```python
from build123d import *

# Parameters (mm, degrees)
BOX018_W               = 5.8
BOX018_H               = 8.7
BOX018_DEPTH           = 4
BOX019_W               = 1.6
BOX019_H               = 3.6
BOX019_DEPTH           = 8.5
BOX016_W               = 3.8
BOX016_H               = 8.5
BOX016_DEPTH           = 9.3
BOX017_W               = 7
BOX017_H               = 12
BOX017_DEPTH           = 9.2
CUT002_ROLL_ANGLE      = 180
CUT002_PLACEMENT_ANGLE = 90
BOX010_W               = 8
BOX010_H               = 3
BOX010_DEPTH           = 2
BOX009_W               = 8
BOX009_H               = 2
BOX009_DEPTH           = 2
BOX011_W               = 8
BOX011_H               = 2
BOX011_DEPTH           = 2
BOX012_W               = 8
BOX012_H               = 3
BOX012_DEPTH           = 2
BOX013_W               = 8
BOX013_H               = 32
BOX013_DEPTH           = 2
BOX014_W               = 15.2
BOX014_H               = 6.6
BOX014_DEPTH           = 4.5
BOX015_W               = 19
BOX015_H               = 10
BOX015_DEPTH           = 5
CUT001_ROLL_ANGLE      = 180
CUT001_PLACEMENT_ANGLE = 90


with BuildPart() as cube017:
    # Box018 → Box018 (new body)
    with BuildSketch(Plane.XY):
        with Locations((2.9, 4.35)):
            Rectangle(BOX018_W, BOX018_H)
    extrude(amount=BOX018_DEPTH)


with BuildPart() as cube018:
    # Box019 → Box019 (new body)
    with BuildSketch(Plane(origin=(1.1, 2.5, 1), x_dir=(1, 0, 0), z_dir=(0, 0, 1))):
        with Locations((0.8, 1.8)):
            Rectangle(BOX019_W, BOX019_H)
    extrude(amount=BOX019_DEPTH)


with BuildPart() as fusion008:
    # Box016 → Box016 (new body)
    with BuildSketch(Plane.XY):
        with Locations((1.9, 4.25)):
            Rectangle(BOX016_W, BOX016_H)
    extrude(amount=BOX016_DEPTH)

    # Fusion008: union Cube017, Cube018
    add(cube017.part)
    add(cube018.part)


with BuildPart() as cut002:
    # Box017 → Box017 (new body)
    with BuildSketch(Plane(origin=(-1.6, -1.65, -0.6), x_dir=(1, 0, 0), z_dir=(0, 0, 1))):
        with Locations((3.5, 6)):
            Rectangle(BOX017_W, BOX017_H)
    extrude(amount=BOX017_DEPTH)

    # Cut002: cut Fusion008
    add(fusion008.part, mode=Mode.SUBTRACT)


with BuildPart() as cut002_1:
    # Cut002 roll: moved
    add(cut002.part.rotate(Axis((0, 0, 0), (1, 0, 0)), CUT002_ROLL_ANGLE))


with BuildPart() as cut002_2:
    # Cut002 placement: moved
    add(cut002_1.part.moved(Location((-0.35, -24.6, 1))).rotate(Axis((-0.35, -24.6, 1), (0, 0, 1)), CUT002_PLACEMENT_ANGLE))


with BuildPart() as cube010:
    # Box010 → Box010 (new body)
    with BuildSketch(Plane(origin=(0, 2.7, 5), x_dir=(1, 0, 0), z_dir=(0, 0, 1))):
        with Locations((4, 1.5)):
            Rectangle(BOX010_W, BOX010_H)
    extrude(amount=BOX010_DEPTH)


with BuildPart() as fusion006:
    # Box009 → Box009 (new body)
    with BuildSketch(Plane(origin=(0, 3.75, 3.5), x_dir=(1, 0, 0), z_dir=(0, 0, 1))):
        with Locations((4, 1)):
            Rectangle(BOX009_W, BOX009_H)
    extrude(amount=BOX009_DEPTH)

    # Fusion006: union Cube010
    add(cube010.part)


with BuildPart() as cube011:
    # Box011 → Box011 (new body)
    with BuildSketch(Plane(origin=(0, -26.3, 3.5), x_dir=(1, 0, 0), z_dir=(0, 0, 1))):
        with Locations((4, 1)):
            Rectangle(BOX011_W, BOX011_H)
    extrude(amount=BOX011_DEPTH)


with BuildPart() as fusion005:
    # Box012 → Box012 (new body)
    with BuildSketch(Plane(origin=(0, -26.3, 5), x_dir=(1, 0, 0), z_dir=(0, 0, 1))):
        with Locations((4, 1.5)):
            Rectangle(BOX012_W, BOX012_H)
    extrude(amount=BOX012_DEPTH)

    # Fusion005: union Cube011
    add(cube011.part)


with BuildPart() as fusion007:
    # Box013 → Box013 (new body)
    with BuildSketch(Plane(origin=(0, -26.3, 1.5), x_dir=(1, 0, 0), z_dir=(0, 0, 1))):
        with Locations((4, 16)):
            Rectangle(BOX013_W, BOX013_H)
    extrude(amount=BOX013_DEPTH)

    # Fusion007: union Fusion006, Fusion005
    add(fusion006.part)
    add(fusion005.part)


with BuildPart() as converter:
    # Box014 → Box014 (new body)
    with BuildSketch(Plane.XY):
        with Locations((7.6, 3.3)):
            Rectangle(BOX014_W, BOX014_H)
    extrude(amount=BOX014_DEPTH)


with BuildPart() as fusion009:
    # Box015 → Box015 (new body)
    with BuildSketch(Plane(origin=(-1.7, -1.5, -1), x_dir=(1, 0, 0), z_dir=(0, 0, 1))):
        with Locations((9.5, 5)):
            Rectangle(BOX015_W, BOX015_H)
    extrude(amount=BOX015_DEPTH)

    # Cut001: cut converter
    add(converter.part, mode=Mode.SUBTRACT)


with BuildPart() as fusion009_1:
    # Cut001 roll: moved
    add(fusion009.part.rotate(Axis((0, 0, 0), (1, 0, 0)), CUT001_ROLL_ANGLE))


with BuildPart() as fusion009_2:
    # Cut001 placement: moved
    add(fusion009_1.part.moved(Location((0.5, -11.7, 0.5))).rotate(Axis((0.5, -11.7, 0.5), (0, 0, 1)), CUT001_PLACEMENT_ANGLE))

    # Fusion009: union Cut002, Fusion007
    add(cut002_2.part)
    add(fusion007.part)


solid = fusion009_2.part
```
For this review, take the finished solid that the model builds, in its own axes (mm). A direction names the side the tool comes from. Coordinates: 2 decimals unless noted, no trailing zeros. Write each loop counter-clockwise with the first axis right and the second up, starting at its lowest first coordinate (ties: lowest second). Pieces come first, ordered by that corner, then holes. Notation, with made-up numbers: (6, 2.25) -> (64, 2.25) arc R30 ccw to (64, 25.25) -> close; hole circle Ø5 at (-22, -22). An arc over 180 degrees is marked (long way). Put each result on its own line as item: value.
Q1. Clearance check with flat-ended pins moving along their axes: pin 1 Ø2 at (x, z) = (4, -1.5) entering from +Y; pin 2 Ø1.2 at (y, z) = (-7.5, -1) entering from +X; pin 3 Ø8 at (y, z) = (-13, -4) entering from -X. State where each tip first meets the part, or that it passes through.
From the geometry:
pin 1: stops at y = 5.6
pin 2: stops at x = 9
pin 3: stops at x = -1
Q2. Take a section at B-B, the plane z = -0.5. State the section outline as (x, y) points, then the cut area to 3 significant figures.
From the geometry:
outline: (-2, -26.2) -> (10, -26.2) -> (10, -19.2) -> (8.35, -19.2) -> (8.35, -24.6) -> (-0.35, -24.6) -> (-0.35, -19.2) -> (-2, -19.2) -> close; (-1, -13.4) -> (9, -13.4) -> (9, 5.6) -> (-1, 5.6) -> close; hole (0.5, -11.7) -> (7.1, -11.7) -> (7.1, 3.5) -> (0.5, 3.5) -> close
area: 127 mm2
Q3. Take a section at D-D, the plane y = -5. State the section outline as (x, z) points, then the cut area to 3 significant figures.
From the geometry:
outline: (-1, -3.5) -> (0.5, -3.5) -> (0.5, 0.5) -> (7.1, 0.5) -> (7.1, -3.5) -> (9, -3.5) -> (9, 1.5) -> (8, 1.5) -> (8, 3.5) -> (0, 3.5) -> (0, 1.5) -> (-1, 1.5) -> close
area: 39.6 mm2
Q4. Take a section at C-C, the plane z = 4.5. State the section outline as (x, y) points, then the cut area to 3 significant figures.
From the geometry:
outline: (0, -26.3) -> (8, -26.3) -> (8, -24.3) -> (0, -24.3) -> close; (0, 3.75) -> (8, 3.75) -> (8, 5.75) -> (0, 5.75) -> close
area: 32.0 mm2
Q5. Tool access review of faces 5 (the flat face through (-0.35, -23, -3)), 6 (the flat face through (7.4, -4, -3.5)), 7 (the flat face through (4, 3, 5)), 8 (the flat face through (0.5, -4, -1)), 9 (the flat face through (-1, -4, -1)): name each direction out of +Z, -Z, +X, -X, +Y, -Y from which nothing blocks a thin tool from reaching the whole face with its end or side.
From the geometry:
face 5: none
face 6: -Z, +X, -X, +Y
face 7: +X, -X
face 8: -Z
face 9: +Z, -Z, -X, +Y
Q6. The part is to be moulded in two halves that separate along X. For faces 1 (the flat face through (4, -4, 0.5)), 2 (the flat face through (0, -10, 3)), 3 (the flat face through (4, -25, 7)), 4 (the flat face through (5, -20, -3)), say which applies: +X half, -X half, draft (parallel to the pull), parting line (faces both ways), or undercut.
From the geometry:
face 1: undercut
face 2: -X half
face 3: draft
face 4: undercut
Q7. Wall thickness on L1, parallel to Y at x = 1, z = -1.25; L2, parallel to Y at x = 5.5, z = -3.25; L3, parallel to X at y = 1.5, z = -2: over which ranges is each line inside the solid? List them lowest first.
From the geometry:
L1: y = -26.2 to -24.6, -13.4 to -11.7, 3.5 to 5.6
L2: y = -26.2 to -24.6, -20.8 to -19.2, -13.4 to -11.7, 3.5 to 5.6
L3: x = -1 to 0.5, 7.1 to 9
